Could you check a few things on this model? Use its own coordinates, in mm. Round coordinates to 2 decimals unless told otherwise and drop trailing zeros. Write each loop counter-clockwise with the first axis right and the second up, starting at its lowest first coordinate (ties: lowest second). Pieces come first, ordered by that corner, then holes. Notation, with made-up numbers: (21, 41.5) -> (51, 41.5) arc R9 ccw to (51, 46.5) -> close; hole circle Ø9 at (88, 80.25). An arc over 180 degrees is marked (long way). Answer as CSV lines item,"result". Start each with the question number.
Q1. If I drill on line 1 (X direction, y = 12, z = 1.25); line 2 (X direction, y = -46, z = 1.95); line 3 (X direction, y = -199, z = 0.9), over which ranges is the centre line in solid material (lowest first)? Write a range as [from, to].
Q2. Will these pins go through, and if not, where does the flat tip stop? pin 1 Ø5 at (x, y) = (-203.5, 0) entering from +Z; pin 2 Ø10.5 at (x, y) = (0, -222.5) entering from +Z; pin 3 Ø1 at (x, z) = (180.5, 0.5) entering from -Y; pin 4 Ø1.5 at (y, z) = (172.5, 1.5) entering from +X.
Q3. Imagine slicing it at C-C on y = -45. Please give me the cut outline in (x, z), and give its area (3 significant figures).
Q4. Imagine slicing it at B-B on x = 12.5. Please give me the cut outline in (y, z).
Q5. Imagine slicing it at D-D on x = 116. Please give me the cut outline in (y, z).
Q6. Imagine slicing it at A-A on z = 1.65. Give the number of separate pieces and of enclosed holes in the cut face, and give its area (3 significant figures).
from build123d import *

# Parameters (mm, degrees)
F0_R     = 237.5
F1_DEPTH = 3
F2_D     = 8
F3_D     = 6


with BuildPart() as f1:
    # F0 (on Top) → F1 (new body)
    with BuildSketch(Plane.XY):
        with BuildLine():
            ThreePointArc((-59, 0), (0, -59), (59, 0))
            ThreePointArc((59, 0), (0, 59), (-59, 0))
        make_face()
        Circle(F0_R)
        with BuildLine():
            ThreePointArc((-59, 0), (0, 59), (59, 0))
            ThreePointArc((59, 0), (0, -59), (-59, 0))
        make_face(mode=Mode.SUBTRACT)
    extrude(amount=F1_DEPTH)

    # F2 (through all)
    with Locations(Plane(origin=(0, 0, 0), x_dir=(1, 0, 0), z_dir=(0, 0, -1))):
        with Locations((222.5, 0), (0, 222.5), (-222.5, 0), (0, -222.5)):
            Hole(F2_D / 2)

    # F3 (through all)
    with Locations(Plane(origin=(0, 0, 0), x_dir=(1, 0, 0), z_dir=(0, 0, -1))):
        with Locations((-203.5, 0), (101.75, 176.23617), (101.75, -176.23617)):
            Hole(F3_D / 2)


solid = f1.part
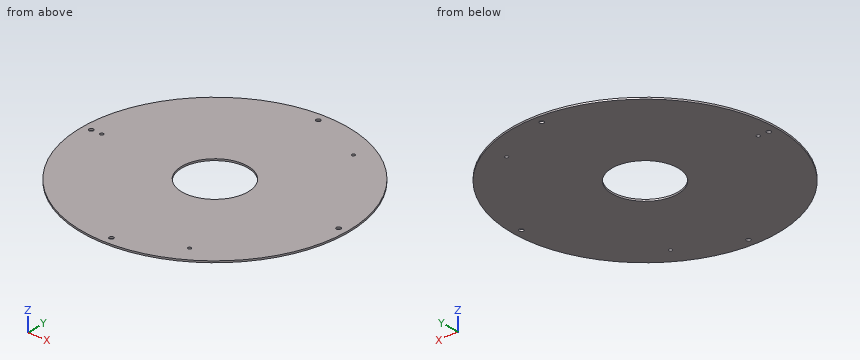
Checks:
1,line 1,"[-237.2, -57.77], [57.77, 237.2]"
1,line 2,"[-233, -36.95], [36.95, 233]"
1,line 3,"[-129.64, 129.64]"
2,pin 1,"through"
2,pin 2,"z = 3"
2,pin 3,"y = -154.94"
2,pin 4,"x = 164.04"
3,outline,"(-233.2, 0) -> (-38.16, 0) -> (-38.16, 3) -> (-233.2, 3) -> close; (38.16, 0) -> (233.2, 0) -> (233.2, 3) -> (38.16, 3) -> close"
3,area,"1,170 mm^2"
4,outline,"(-237.17, 0) -> (-57.66, 0) -> (-57.66, 3) -> (-237.17, 3) -> close; (57.66, 0) -> (237.17, 0) -> (237.17, 3) -> (57.66, 3) -> close"
5,outline,"(-207.24, 0) -> (207.24, 0) -> (207.24, 3) -> (-207.24, 3) -> close"
6,separate pieces,"1"
6,enclosed holes,"8"
6,area,"166,000 mm^2"
